Verification items for the finished model (mm, model axes). Face numbers are marked on the shaded views. A direction names the side the tool comes from. Round coordinates to 2 decimals unless told otherwise and drop trailing zeros. Order: outer loops, then holes, each group sorted by start corner. A loop starts at its lowest first (then second) coordinate and runs counter-clockwise, first axis right, second up.
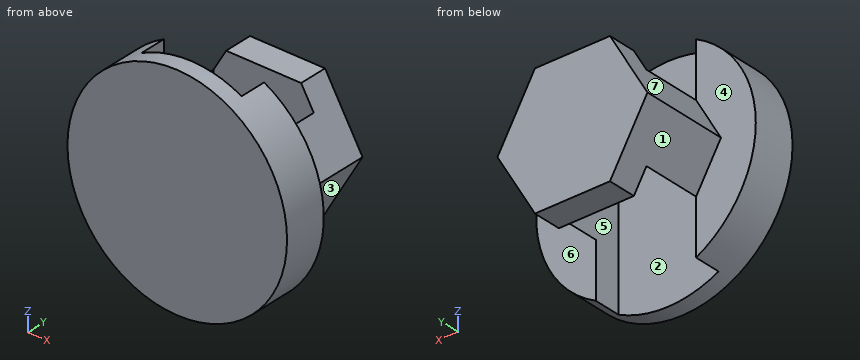
Autodesk Inventor part; units mm, degrees
ref_plane "YZ Plane" through (0, 0, 0) normal (1, 0, 0) x (0, 1, 0)
ref_plane "XZ Plane" through (0, 0, 0) normal (0, 1, 0) x (-1, 0, 0)
ref_plane "XY Plane" through (0, 0, 0) normal (0, 0, 1) x (1, 0, 0)
sketch "Эскиз1" plane through (0, 0, 0) normal (0, 1, 0) x (-1, 0, 0)
  circle A0 centre (0, 0) radius 50
  dimension "d0" = 100
extrude "Выдавливание1" add sketch "Эскиз1" along normal blind 20
sketch "Эскиз2" plane through (0, 20, 0) normal (0, 1, 0) x (1, 0, 0)
  line L0 (17.0801, 29.5836) -> (34.1603, 0)
  line L1 (34.1603, 0) -> (17.0801, -29.5836)
  line L2 (17.0801, -29.5836) -> (-17.0801, -29.5836)
  line L3 (-17.0801, -29.5836) -> (-34.1603, 0)
  line L4 (-34.1603, 0) -> (-17.0801, 29.5836)
  line L5 (-17.0801, 29.5836) -> (17.0801, 29.5836)
  point P0 (0, 0)
  point P1 (0, 0)
extrude "Выдавливание2" add sketch "Эскиз2" along normal blind 40
sketch "Эскиз3" plane through (0, 0, 0) normal (0, 0, 1) x (1, 0, 0)
  line L0 (-22.8201, 7.7625) -> (22.8201, 7.7625)
  line L1 (22.8201, 7.7625) -> (22.8201, 46.9937)
  line L2 (22.8201, 46.9937) -> (-22.8201, 46.9937)
  line L3 (-22.8201, 46.9937) -> (-22.8201, 7.7625)
  line L4 (-22.8201, 7.7625) -> (22.8201, 46.9937) construction
  line L5 (22.8201, 7.7625) -> (-22.8201, 46.9937) construction
  point P0 (0, 0)
  point P1 (0, 27.3781)
extrude "Выдавливание3" cut sketch "Эскиз3" against normal through all both and the other way through all
sketch "Эскиз4" plane through (0, 0, 0) normal (1, 0, 0) x (0, 1, 0)
  point P0 (0, 0)
1) Sectioned sample at A-A on x = 0. Record the cut outline in (y, z).
2) Scan lines: probe 1 along Y at (x, z) = (17, 16); probe 2 along Y at (x, z) = (-41.5, -27); probe 3 along Y at (x, z) = (-6.5, 41). Record each from-to range of solid material in increasing order.
3) Go/stop test with flat-tipped pins: pin 1 Ø12 at (y, z) = (27, -7) entering from +X; pin 2 Ø8 at (x, z) = (42.5, 20) entering from +Y; pin 3 Ø4 at (y, z) = (10, -19.5) entering from -X; pin 4 Ø12 at (x, z) = (-3, 33.5) entering from +Y. Record where each tip stops, or that it passes through.
4) Sectioned sample at C-C on y = 49. Record the cut outline in (x, z).
5) Tool access check on the marked faces 5, 6 and 7. Record the directions out of +Z, -Z, +X, -X, +Y, -Y that give a thin tool (end or side, any length) a straight path to the whole face; none if there is none.
6) Sectioned sample at D-D on z = -41. Record the cut outline in (x, y), then the cut area to 3 significant figures.
7) Sectioned sample at B-B on z = 14. Record the cut outline in (x, y).
8) Draft check along X on the marked faces 1, 2, 3 and 4. Enter one of: released by +X, released by -X, zero draft, split by the parting line, or undercut.
Returned:
1. outline: (0, -50) - (7.76, -50) - (7.76, 50) - (0, 50) - close; (46.99, -29.58) - (60, -29.58) - (60, 29.58) - (46.99, 29.58) - close
2. probe 1: y = 0 to 7.76, 46.99 to 60
2. probe 2: y = 0 to 20
2. probe 3: y = 0 to 7.76
3. pin 1: stops at x = 33.58
3. pin 2: stops at y = 20
3. pin 3: stops at x = -46.84
3. pin 4: stops at y = 60
4. outline: (-34.16, 0) - (-17.08, -29.58) - (17.08, -29.58) - (34.16, 0) - (17.08, 29.58) - (-17.08, 29.58) - close
5. face 5: +Z, -Z
5. face 6: +X, +Y
5. face 7: +Z, -X, +Y
6. outline: (-28.62, 0) - (28.62, 0) - (28.62, 20) - (22.82, 20) - (22.82, 7.76) - (-22.82, 7.76) - (-22.82, 20) - (-28.62, 20) - close
6. area: 586 mm2
7. outline: (-48, 0) - (48, 0) - (48, 20) - (26.08, 20) - (26.08, 60) - (-26.08, 60) - (-26.08, 20) - (-48, 20) - close; hole (-22.82, 7.76) - (22.82, 7.76) - (22.82, 46.99) - (-22.82, 46.99) - close
8. face 1: released by -X
8. face 2: undercut
8. face 3: released by +X
8. face 4: zero draft
